from build123d import *

# Parameters (mm, degrees)
F0_W     = 127
F0_H     = 76.2
F1_DEPTH = 25.4
F2_W     = 120.65
F2_H     = 69.85
F3_DEPTH = 22.225
F4_R     = 1.5748


with BuildPart() as f1:
    # F0 (on Top) → F1 (new body)
    with BuildSketch(Plane.XY):
        with Locations((6.366314, 2.805781)):
            Rectangle(F0_W, F0_H)
    extrude(amount=-F1_DEPTH)

    # F2 (on face) → F3 (cut)
    with BuildSketch(Plane.XY):
        with Locations((6.366314, 2.805781)):
            Rectangle(F2_W, F2_H)
    extrude(amount=-F3_DEPTH, mode=Mode.SUBTRACT)

    # F4
    f4_edges = [f1.edges().sort_by_distance(p)[0] for p in [
        (-57.133686, 2.805781, 0),
        (6.366314, -35.294219, 0),
        (69.866314, 2.805781, 0),
        (6.366314, 40.905781, 0),
        (6.366314, 37.730781, 0),
        (-53.958686, 2.805781, 0),
        (6.366314, -32.119219, 0),
        (66.691314, 2.805781, 0),
        (69.866314, -35.294219, -12.7),
        (-57.133686, -35.294219, -12.7),
        (6.366314, -35.294219, -25.4),
        (69.866314, 2.805781, -25.4),
        (69.866314, 40.905781, -12.7),
        (-57.133686, 40.905781, -12.7),
        (6.366314, 40.905781, -25.4),
        (-57.133686, 2.805781, -25.4),
    ]]
    fillet(f4_edges, radius=F4_R)


solid = f1.part
Verification items for the finished model (mm, model axes). A direction names the side the tool comes from. Round coordinates to 2 decimals unless told otherwise and drop trailing zeros. Loops run counter-clockwise (first coordinate to the right, second up) from the corner with the lowest first, then second, coordinate; pieces in that order, holes last. Notation, with made-up numbers: (18, 58) - (31, 58) arc R13 cw to (31, 78) - close; hole circle Ø8 at (-19, -22.5). An arc over 180 degrees is marked (long way). Use a Markdown table: item, result. Add a question column.
1. Thickness scan on probe 1 along X at (y, z) = (-31, -5.25); probe 2 along Y at (x, z) = (-18.5, -14); probe 3 along Z at (x, y) = (49.5, 2) (3 decimals). Record the ranges inside material, lowest first. Write a range as [from, to].
2. Release check for a two-part mould opening along X. For faces 3 (the face through (5, -35.294, -13)), 4 (the face through (69.866, 2, -13)), 5 (the face through (-57.134, 2, -13)), 6 (the face through (6, 37.731, -12)) record: released by +X, released by -X, zero draft, split by the parting line, or undercut.
3. Section check B-B, the plane x = -4. Record the boundary of the cut face in (y, z) (3 decimals).
4. Access from +Z, -Z, +X, -X, +Y, -Y to the whole of each face (thin tool, end or side, straight path). Record for faces 1 (the face through (6, 3, -22.225)), 2 (the face through (5, 3, -25.4)).
5. Section check A-A, the plane z = -6. Record the boundary of the cut face in (x, y), plus the area to 3 significant figures.
6. Gauge pin test, flat end, axial feed: pin 1 (1 mm diameter, centred on x = -27.5, y = -2.5, fed in from +Z) (3 decimals). Record the tip position at first contact, or that the pin passes through.
7. Section check C-C, the plane y = -14.5. Record the boundary of the cut face in (x, z) (3 decimals), plus the area to 3 significant figures.
Checks:
| question | item | result |
|---|---|---|
| 1 | probe 1 | x = [-57.13, -53.96], [66.69, 69.87] |
| 1 | probe 2 | y = [-35.29, -32.12], [37.73, 40.91] |
| 1 | probe 3 | z = [-25.4, -22.225] |
| 2 | face 3 | zero draft |
| 2 | face 4 | released by +X |
| 2 | face 5 | released by -X |
| 2 | face 6 | undercut |
| 3 | outline | (-35.294, -23.825) arc R1.575 ccw to (-33.719, -25.4) - (39.331, -25.4) arc R1.575 ccw to (40.906, -23.825) - (40.906, -1.575) arc R1.575 ccw to (39.331, 0) - (39.306, 0) arc R1.575 ccw to (37.731, -1.575) - (37.731, -22.225) - (-32.119, -22.225) - (-32.119, -1.575) arc R1.575 ccw to (-33.694, 0) - (-33.719, 0) arc R1.575 ccw to (-35.294, -1.575) - close |
| 4 | face 1 | +Z |
| 4 | face 2 | -Z, +X, -X, +Y, -Y |
| 5 | outline | (-57.13, -33.72) arc R1.57 ccw to (-55.56, -35.29) - (68.29, -35.29) arc R1.57 ccw to (69.87, -33.72) - (69.87, 39.33) arc R1.57 ccw to (68.29, 40.91) - (-55.56, 40.91) arc R1.57 ccw to (-57.13, 39.33) - close; hole (-53.96, -32.12) - (66.69, -32.12) - (66.69, 37.73) - (-53.96, 37.73) - close |
| 5 | area | 1,250 mm^2 |
| 6 | pin 1 | stops at z = -22.225 |
| 7 | outline | (-57.134, -23.825) arc R1.575 ccw to (-55.559, -25.4) - (68.292, -25.4) arc R1.575 ccw to (69.866, -23.825) - (69.866, -1.575) arc R1.575 ccw to (68.292, 0) - (68.266, 0) arc R1.575 ccw to (66.691, -1.575) - (66.691, -22.225) - (-53.959, -22.225) - (-53.959, -1.575) arc R1.575 ccw to (-55.533, 0) - (-55.559, 0) arc R1.575 ccw to (-57.134, -1.575) - close |
| 7 | area | 541 mm^2 |
